Verification items for the finished model (mm, model axes). Face numbers are marked on the shaded views. A direction names the side the tool comes from. Coordinates: 2 decimals unless noted, no trailing zeros. Loops run counter-clockwise (first coordinate to the right, second up) from the corner with the lowest first, then second, coordinate; pieces in that order, holes last. Notation, with made-up numbers: (85, 43.5) -> (103, 43.5) arc R23 cw to (103, 74.5) -> close; hole circle Ø2 at (2.5, -26.5). An arc over 180 degrees is marked (long way). Answer as a JSON object with one key per item and string values. Group by question number.
Q1. Release check for a two-part mould opening along Y. For the marked faces 1, 2 and 3 record: released by +Y, released by -Y, zero draft, split by the parting line, or undercut.
Q2. Set-up check for the marked faces 4 and 5: record each of +Z, -Z, +X, -X, +Y, -Y from which the full face is reachable in a straight line by a thin tool's end or side.
Q3. Gauge pin test, flat ends, axial feed: pin 1 Ø2 at (x, y) = (-26.5, 39.5) entering from +Z (3 decimals); pin 2 Ø5 at (x, z) = (23, 5) entering from -Y; pin 3 Ø4 at (x, z) = (-5.5, 13.5) entering from -Y. Record the tip position at first contact, or that the pin passes through.
Q4. Scan lines: L1, parallel to Z at x = -18.5, y = 19.5 (3 decimals); L2, parallel to Z at x = 42.5, y = -21.5 (3 decimals); L3, parallel to Y at x = 1, z = 13.5. Record each from-to range of solid material in increasing order.
Q5. Cross-section at C-C on z = 14. Record the boundary of the cut face in (x, y) (1 decimal), and give its area (3 significant figures).
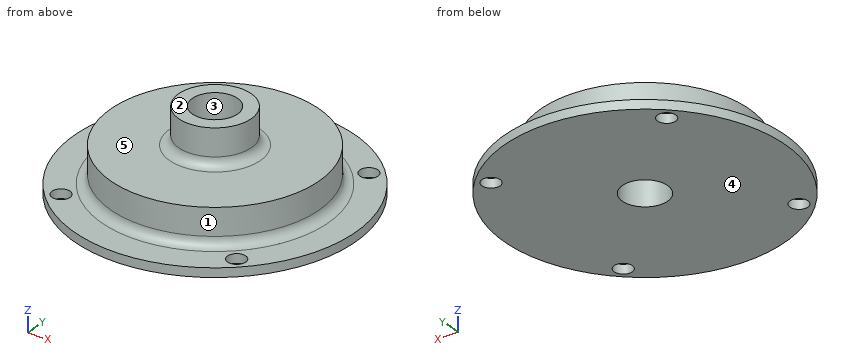
```python
from build123d import *

# Parameters (mm, degrees)
SKETCH1_R           = 49.2125
SKETCH1_R_2         = 3.175
BASE_EXTRUDE_DEPTH  = 3.175
SKETCH2_R           = 36.5125
BOSS_EXTRUDE1_DEPTH = 12.7
SKETCH3_R           = 12.7
BOSS_EXTRUDE2_DEPTH = 12.7
FILLET1_R           = 3.175
SKETCH4_R           = 7.9375
CUT_EXTRUDE1_DEPTH  = 76.23477213


with BuildPart() as part:
    # Sketch1 → Base-Extrude (new body)
    with BuildSketch(Plane.XY):
        Circle(SKETCH1_R)
        with Locations((31.430896424, 31.430896424)):
            Circle(SKETCH1_R_2, mode=Mode.SUBTRACT)
        with Locations((-31.430896424, -31.430896424)):
            Circle(SKETCH1_R_2, mode=Mode.SUBTRACT)
        with Locations((31.430896424, -31.430896424)):
            Circle(SKETCH1_R_2, mode=Mode.SUBTRACT)
        with Locations((-31.430896424, 31.430896424)):
            Circle(SKETCH1_R_2, mode=Mode.SUBTRACT)
    extrude(amount=BASE_EXTRUDE_DEPTH)

    # Sketch2 → Boss-Extrude1 (add)
    with BuildSketch(Plane.XY.offset(3.175)):
        Circle(SKETCH2_R)
    extrude(amount=BOSS_EXTRUDE1_DEPTH)

    # Sketch3 → Boss-Extrude2 (add)
    with BuildSketch(Plane.XY.offset(15.875)):
        Circle(SKETCH3_R)
    extrude(amount=BOSS_EXTRUDE2_DEPTH)

    # Fillet1
    fillet1_edges = [part.edges().sort_by_distance(p)[0] for p in [
        (-36.5125, 0, 3.175),
        (-12.7, 0, 15.875),
    ]]
    fillet(fillet1_edges, radius=FILLET1_R)

    # Sketch4 → Cut-Extrude1 (cut, through all)
    with BuildSketch(Plane.XY.offset(28.575)):
        Circle(SKETCH4_R)
    extrude(amount=-CUT_EXTRUDE1_DEPTH, mode=Mode.SUBTRACT)


solid = part.part
```
Computed values:
{
 "1": {"face 1": "split by the parting line", "face 2": "zero draft", "face 3": "undercut"},
 "2": {"face 4": "-Z, +X, -X, +Y, -Y", "face 5": "+Z"},
 "3": {"pin 1": "stops at z = 3.175", "pin 2": "stops at y = -44.37", "pin 3": "stops at y = -36.34"},
 "4": {"L1": "z = 0 to 15.875", "L2": "z = 0 to 3.175", "L3": "y = -36.5 to -7.87, 7.87 to 36.5"},
 "5": {"outline": "circle Ø73 at (0, 0); hole circle Ø15.9 at (0, 0)", "area": "3,990 mm²"}
}
